Could you check a few things on this model? Use its own coordinates, in mm. Give positions to 0.01 mm unless a question says otherwise; leave off trailing zeros. Use one line per item in the form item = value.
from build123d import *

# Parameters (mm, degrees)
CROQUIS1_R              = 6
CROQUIS1_R_2            = 3
CROQUIS1_R_3            = 1.5
SALIENTE_EXTRUIR1_DEPTH = 5
REDONDEO1_R             = 5


with BuildPart() as part:
    # Croquis1 → Saliente-Extruir1 (new body)
    with BuildSketch(Plane.XY):
        with BuildLine():
            Line((100, 0), (100, -49))
            ThreePointArc((100, -49), (97.656854249, -54.656854249), (92, -57))
            Line((92, -57), (-92, -57))
            ThreePointArc((-92, -57), (-97.656854249, -54.656854249), (-100, -49))
            Line((-100, -49), (-100, 0))
            Line((-100, 0), (-100, 5))
            Line((-100, 5), (100, 5))
            Line((100, 5), (100, 0))
        make_face()
        with Locations((0, -27)):
            Circle(CROQUIS1_R, mode=Mode.SUBTRACT)
        with Locations((72, -19.25)):
            Circle(CROQUIS1_R_2, mode=Mode.SUBTRACT)
        with Locations((-72, -19.25)):
            Circle(CROQUIS1_R_2, mode=Mode.SUBTRACT)
        with Locations((72, -39.25)):
            Circle(CROQUIS1_R_3, mode=Mode.SUBTRACT)
        with Locations((52, -19.25)):
            Circle(CROQUIS1_R_3, mode=Mode.SUBTRACT)
        with Locations((92, -19.25)):
            Circle(CROQUIS1_R_3, mode=Mode.SUBTRACT)
        with Locations((-72, -39.25)):
            Circle(CROQUIS1_R_3, mode=Mode.SUBTRACT)
        with Locations((-92, -19.25)):
            Circle(CROQUIS1_R_3, mode=Mode.SUBTRACT)
        with Locations((-52, -19.25)):
            Circle(CROQUIS1_R_3, mode=Mode.SUBTRACT)
        with Locations((15, -45)):
            Circle(CROQUIS1_R_3, mode=Mode.SUBTRACT)
        with Locations((35, -45)):
            Circle(CROQUIS1_R_3, mode=Mode.SUBTRACT)
        with Locations((-35, -45)):
            Circle(CROQUIS1_R_3, mode=Mode.SUBTRACT)
        with Locations((-15, -45)):
            Circle(CROQUIS1_R_3, mode=Mode.SUBTRACT)
        with Locations((-15, -27)):
            Circle(CROQUIS1_R_3, mode=Mode.SUBTRACT)
        with Locations((15, -27)):
            Circle(CROQUIS1_R_3, mode=Mode.SUBTRACT)
        with Locations((0, -37)):
            Circle(CROQUIS1_R_3, mode=Mode.SUBTRACT)
    extrude(amount=SALIENTE_EXTRUIR1_DEPTH)

    # Redondeo1
    redondeo1_edges = [part.edges().sort_by_distance(p)[0] for p in [
        (-100, 5, 2.5),
        (100, 5, 2.5),
    ]]
    fillet(redondeo1_edges, radius=REDONDEO1_R)


solid = part.part
1) If I drill on L1, parallel to X at y = -39, z = 1.3; L2, parallel to Y at x = 72, z = 2.7; L3, parallel to Y at x = 15, z = 2.8, over which ranges is the centre line in solid material (lowest first)?
Checked values:
L1 = -100 to -73.48, -70.52 to 70.52, 73.48 to 100
L2 = -57 to -40.75, -37.75 to -22.25, -16.25 to 5
L3 = -57 to -46.5, -43.5 to -28.5, -25.5 to 5
2) I want a section at A-A, the plane z = 1.5. Count the separate pieces of the cut face and the enclosed holes in it, plus the area to 3 significant figures.
Checked values:
separate_pieces = 1
enclosed_holes = 16
area = 12,100 mm2
3) Thinking about a two-plate mould opening in Y: for faces 1 (the cylindrical face through (-1.301, -32.857, 2.465)), 2 (the flat face through (1, -57, 2)), 3 (the cylindrical face through (-74.381, -21.075, 2.465)), 4 (the flat face through (100, -24, 2)), which applies, released by +Y, released by -Y, zero draft, split by the parting line, or undercut?
Checked values:
face_1 = undercut
face_2 = released by -Y
face_3 = undercut
face_4 = zero draft
4) For pin 1 Ø4 at (x, y) = (-92, -19.25) entering from +Z, with a flat end and sliding along its axis, tell me the tip position at first contact or that it passes through.
Checked values:
pin_1 = 5
